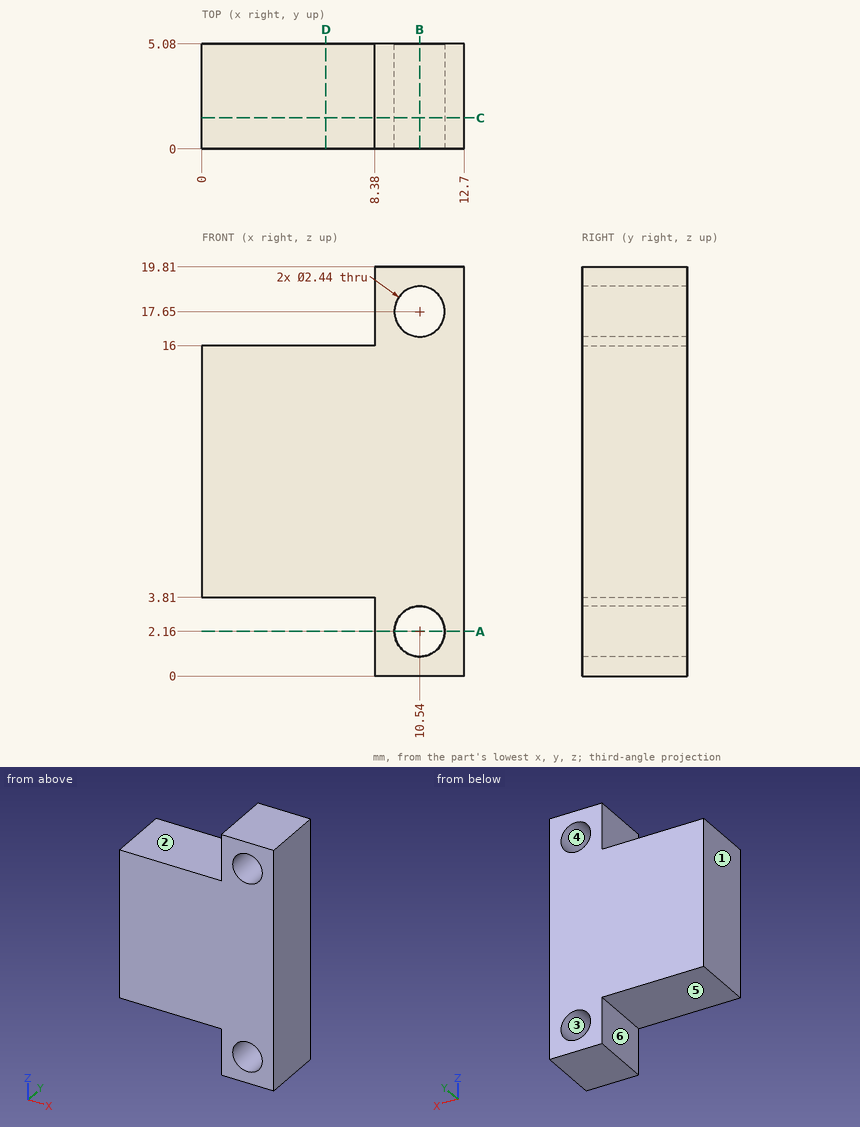
Study the drawing (mm; zero at the part's minimum x, y, z) and answer. A direction names the side the tool comes from. Give positions to 0.01 mm unless a question says otherwise; leave off trailing zeros. Write each loop counter-clockwise with the first axis right and the second up, starting at its lowest first coordinate (ties: lowest second). Pieces come first, ordered by that corner, then holes.
Item 1: Section D-D, the plane x = 6 is taken. Write down the section's boundary in (y, z), plus the area to 3 significant figures.
Item 2: Section C-C, the plane y = 1.5 is taken. Write down the section's boundary in (x, z).
Item 3: Section B-B, the plane x = 10.54 is taken. Write down the section's boundary in (y, z).
Item 4: Which of the six approach directions +Z, -Z, +X, -X, +Y, -Y give full straight-line access (tool end or side, diameter ignored) to the marked faces 1 and 2?
Item 5: Flat-ended cylindrical pins translate along their axes: P1, Ø1, axis at x = 7, y = 2, coming from the -Z side; P2, Ø1.9, axis at y = 3, z = 1.5, coming from the -X side. Find the tip coordinate at first contact, or state that the pin passes through.
Item 6: Determine the mould class of the marked faces 3, 4, 5 and 6 for opening direction X: released by +X, released by -X, zero draft, split by the parting line, or undercut.
Item 7: Find the intervals of material crossed by line 1 along Z through (x, y) = (10.54, 1.1); line 2 along X through (y, z) = (2.2, 2.16); line 3 along X through (y, z) = (2.5, 16.25), in increasing order.
Item 8: Section A-A, the plane z = 2.16 is taken. Write down the section's boundary in (x, y).
Completed:
1. outline: (0, 3.81) - (5.08, 3.81) - (5.08, 16) - (0, 16) - close
1. area: 61.9 mm2
2. outline: (0, 3.81) - (8.38, 3.81) - (8.38, 0) - (12.7, 0) - (12.7, 19.81) - (8.38, 19.81) - (8.38, 16) - (0, 16) - close; hole circle Ø2.44 at (10.54, 2.16); hole circle Ø2.44 at (10.54, 17.65)
3. outline: (0, 0) - (5.08, 0) - (5.08, 0.94) - (0, 0.94) - close; (0, 3.38) - (5.08, 3.38) - (5.08, 16.43) - (0, 16.43) - close; (0, 18.87) - (5.08, 18.87) - (5.08, 19.81) - (0, 19.81) - close
4. face 1: +Z, -Z, -X, +Y, -Y
4. face 2: +Z, -X, +Y, -Y
5. P1: stops at z = 3.81
5. P2: stops at x = 8.38
6. face 3: undercut
6. face 4: undercut
6. face 5: zero draft
6. face 6: released by -X
7. line 1: z = 0 to 0.94, 3.38 to 16.43, 18.87 to 19.81
7. line 2: x = 8.38 to 9.32, 11.76 to 12.7
7. line 3: x = 8.38 to 12.7
8. outline: (8.38, 0) - (9.32, 0) - (9.32, 5.08) - (8.38, 5.08) - close; (11.76, 0) - (12.7, 0) - (12.7, 5.08) - (11.76, 5.08) - close
